Geometry check sheet. Reference: drawing and pictorial views, mm from the part's lowest x, y, z. A direction names the side the tool comes from. Round coordinates to 2 decimals unless told otherwise and drop trailing zeros. Order: outer loops, then holes, each group sorted by start corner. A loop starts at its lowest first (then second) coordinate and runs counter-clockwise, first axis right, second up.
Q1. Depth check by flat-ended pin: P1, Ø2.5, axis at x = 127.5, y = 64.5, coming from the +Z side; P2, Ø1, axis at x = 71.5, z = 0.5, coming from the +Y side; P3, Ø1.6, axis at x = 118.5, z = 0.5, coming from the -Y side. Enter the tip coordinate at first touch or a pass-through.
Q2. Cross-section at A-A on z = 2.9. Record the cut outline in (x, y).
Q3. Cross-section at C-C on x = 37. Record the cut outline in (y, z).
Q4. Scan lines: probe 1 along Y at (x, z) = (127.5, 0.85); probe 2 along X at (y, z) = (48.5, 3.55); probe 3 along X at (y, z) = (64.5, 1.1). Record each from-to range of solid material in increasing order.
Q5. Cross-section at B-B on y = 42.5. Record the cut outline in (x, z), then the cut area to 3 significant figures.
Q6. Set-up check for the marked faces 3, 4 and 5: record each of +Z, -Z, +X, -X, +Y, -Y from which the full face is reachable in a straight line by a thin tool's end or side.
Q7. Mould release check, pull along X, two halves, no side actions. Record for the marked faces 1 and 2: +X half, -X half, draft (parallel to the pull), parting line (faces both ways), or undercut.
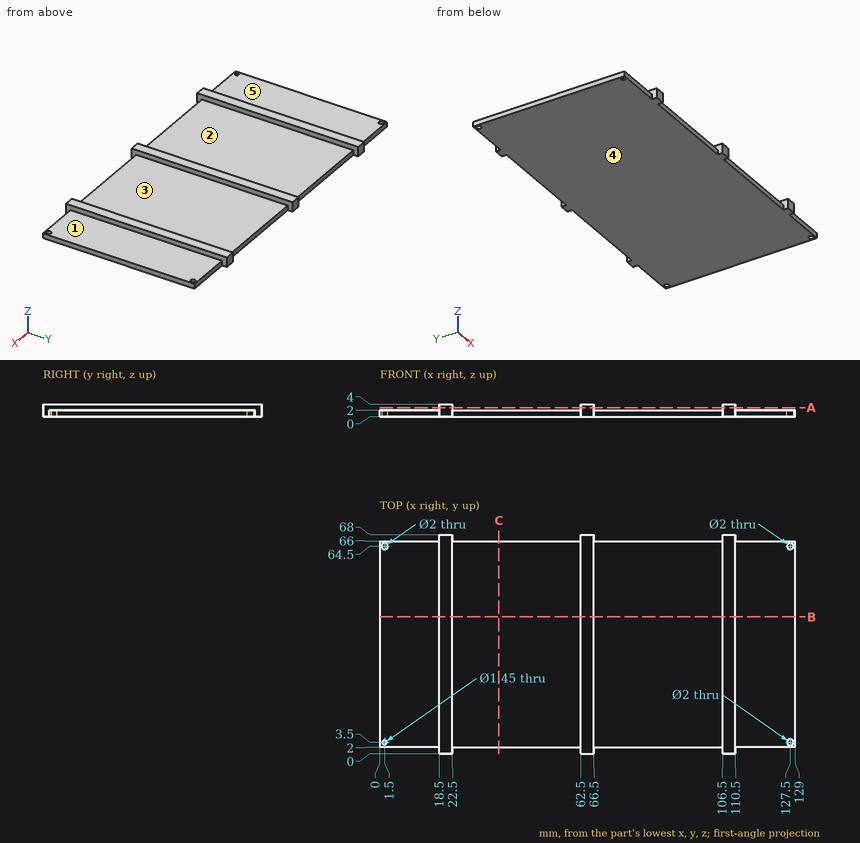
Results found:
1. P1: stops at z = 2
1. P2: stops at y = 66
1. P3: stops at y = 2
2. outline: (18.5, 0) - (22.5, 0) - (22.5, 68) - (18.5, 68) - close; (62.5, 0) - (66.5, 0) - (66.5, 68) - (62.5, 68) - close; (106.5, 0) - (110.5, 0) - (110.5, 68) - (106.5, 68) - close
3. outline: (2, 0) - (66, 0) - (66, 2) - (2, 2) - close
4. probe 1: y = 2 to 2.5, 4.5 to 63.5, 65.5 to 66
4. probe 2: x = 18.5 to 22.5, 62.5 to 66.5, 106.5 to 110.5
4. probe 3: x = 0 to 0.5, 2.5 to 126.5, 128.5 to 129
5. outline: (0, 0) - (129, 0) - (129, 2) - (110.5, 2) - (110.5, 4) - (106.5, 4) - (106.5, 2) - (66.5, 2) - (66.5, 4) - (62.5, 4) - (62.5, 2) - (22.5, 2) - (22.5, 4) - (18.5, 4) - (18.5, 2) - (0, 2) - close
5. area: 282 mm2
6. face 3: +Z, +Y, -Y
6. face 4: -Z, +X, -X, +Y, -Y
6. face 5: +Z, -X, +Y, -Y
7. face 1: draft
7. face 2: undercut
